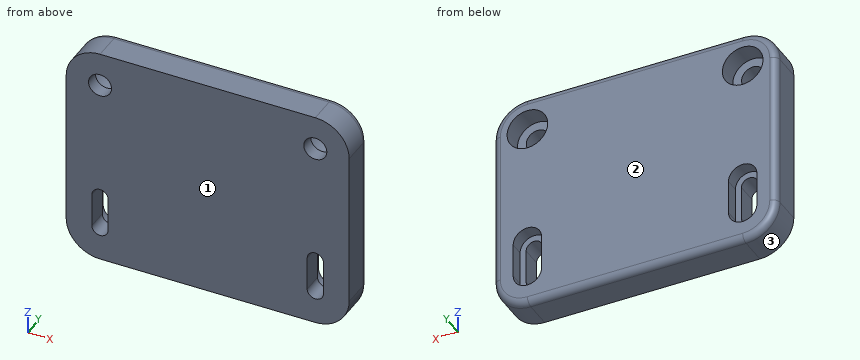
```python
from build123d import *

# Parameters (mm, degrees)
SKETCH1_W           = 41.8
SKETCH1_H           = 33
SKETCH1_R           = 1.7
BOSS_EXTRUDE1_DEPTH = 5
FILLET1_R           = 5
FILLET2_R           = 1
SKETCH2_R           = 3
SKETCH2_R_2         = 1.7
CUT_EXTRUDE1_DEPTH  = 3
CUT_EXTRUDE2_DEPTH  = 2


with BuildPart() as part:
    # Sketch1 → Boss-Extrude1 (new body)
    with BuildSketch(Plane(origin=(0, 0, 0), x_dir=(1, 0, 0), z_dir=(0, 1, 0))):
        with Locations((20.9, 16.5)):
            Rectangle(SKETCH1_W, SKETCH1_H)
        with Locations((5, 5)):
            Circle(SKETCH1_R, mode=Mode.SUBTRACT)
        with Locations((36.8, 5)):
            Circle(SKETCH1_R, mode=Mode.SUBTRACT)
        with BuildLine():
            Line((3.8, 23), (3.8, 28))
            ThreePointArc((3.8, 28), (5, 29.2), (6.2, 28))
            Line((6.2, 28), (6.2, 23))
            ThreePointArc((6.2, 23), (5, 21.8), (3.8, 23))
        make_face(mode=Mode.SUBTRACT)
        with BuildLine():
            Line((35.6, 23), (35.6, 28))
            ThreePointArc((35.6, 28), (36.8, 29.2), (38, 28))
            Line((38, 28), (38, 23))
            ThreePointArc((38, 23), (36.8, 21.8), (35.6, 23))
        make_face(mode=Mode.SUBTRACT)
    extrude(amount=BOSS_EXTRUDE1_DEPTH)

    # Fillet1
    fillet1_edges = [part.edges().sort_by_distance(p)[0] for p in [
        (0, 2.5, -33),
        (41.8, 2.5, -33),
        (41.8, 2.5, 0),
        (0, 2.5, 0),
    ]]
    fillet(fillet1_edges, radius=FILLET1_R)

    # Fillet2
    fillet2_edges = [part.edges().sort_by_distance(p)[0] for p in [
        (0, 5, -16.5),
        (20.9, 5, -33),
        (20.9, 5, 0),
        (41.8, 5, -16.5),
        (1.464466094, 5, -1.464466094),
        (40.335533906, 5, -1.464466094),
        (40.335533906, 5, -31.535533906),
        (1.464466094, 5, -31.535533906),
    ]]
    fillet(fillet2_edges, radius=FILLET2_R)

    # Sketch2 → Cut-Extrude1 (cut)
    with BuildSketch(Plane(origin=(0, 5, 0), x_dir=(1, 0, 0), z_dir=(0, 1, 0))):
        with Locations((5, 5)):
            Circle(SKETCH2_R)
        with Locations((5, 5)):
            Circle(SKETCH2_R_2, mode=Mode.SUBTRACT)
        with Locations((36.8, 5)):
            Circle(SKETCH2_R)
        with Locations((36.8, 5)):
            Circle(SKETCH2_R_2, mode=Mode.SUBTRACT)
    extrude(amount=-CUT_EXTRUDE1_DEPTH, mode=Mode.SUBTRACT)

    # Sketch2_3 → Cut-Extrude2 (cut)
    with BuildSketch(Plane(origin=(0, 5, 0), x_dir=(1, 0, 0), z_dir=(0, 1, 0))):
        with BuildLine():
            Line((2.9, 28), (2.9, 23))
            ThreePointArc((2.9, 23), (5, 20.9), (7.1, 23))
            Line((7.1, 23), (7.1, 28))
            ThreePointArc((7.1, 28), (5, 30.1), (2.9, 28))
        make_face()
        with BuildLine():
            Line((6.2, 28), (6.2, 23))
            ThreePointArc((6.2, 23), (5, 21.8), (3.8, 23))
            Line((3.8, 23), (3.8, 28))
            ThreePointArc((3.8, 28), (5, 29.2), (6.2, 28))
        make_face(mode=Mode.SUBTRACT)
        with BuildLine():
            Line((34.7, 28), (34.7, 23))
            ThreePointArc((34.7, 23), (36.8, 20.9), (38.9, 23))
            Line((38.9, 23), (38.9, 28))
            ThreePointArc((38.9, 28), (36.8, 30.1), (34.7, 28))
        make_face()
        with BuildLine():
            Line((38, 28), (38, 23))
            ThreePointArc((38, 23), (36.8, 21.8), (35.6, 23))
            Line((35.6, 23), (35.6, 28))
            ThreePointArc((35.6, 28), (36.8, 29.2), (38, 28))
        make_face(mode=Mode.SUBTRACT)
    extrude(amount=-CUT_EXTRUDE2_DEPTH, mode=Mode.SUBTRACT)


solid = part.part
```
Build history of the part. All positions in model axes, mm. Face numbers are marked on the shaded views. Round coordinates to 2 decimals unless told otherwise and drop trailing zeros. Write each loop counter-clockwise with the first axis right and the second up, starting at its lowest first coordinate (ties: lowest second). Pieces come first, ordered by that corner, then holes.
1) Drill centre lines: probe 1 along Z at (x, y) = (36.8, 3.65); probe 2 along Z at (x, y) = (5, 1.05); probe 3 along X at (y, z) = (2.35, -28.5). Where is each one in solid material? Low to high.
2) Pin check, flat tip, straight feed: pin 1 (5.5 mm diameter, centred on x = 5, z = -5, fed in from +Y). Stop position of the tip, or through.
3) Mould opens along Y. For the marked faces 1, 2 and 3 say: +Y half, -Y half, draft (parallel to the pull), parting line (faces both ways), or undercut.
4) Band-saw the part on B-B, the plane z = -23.5. List the corners of the cut face in (x, y), and give its area (3 significant figures).
5) Band-saw the part on A-A, the plane y = 1.3. List the corners of the cut face in (x, z).
Ans:
1. probe 1: z = -33 to -30.1, -20.9 to -8, -2 to 0
1. probe 2: z = -33 to -29.2, -21.8 to -6.7, -3.3 to 0
1. probe 3: x = 0.03 to 3.91, 6.09 to 35.71, 37.89 to 41.77
2. pin 1: stops at y = 2
3. face 1: -Y half
3. face 2: +Y half
3. face 3: draft
4. outline: (0, 0) - (3.8, 0) - (3.8, 3) - (2.9, 3) - (2.9, 5) - (1, 5) arc R1 ccw to (0, 4) - close; (6.2, 0) - (35.6, 0) - (35.6, 3) - (34.7, 3) - (34.7, 5) - (7.1, 5) - (7.1, 3) - (6.2, 3) - close; (38, 0) - (41.8, 0) - (41.8, 4) arc R1 ccw to (40.8, 5) - (38.9, 5) - (38.9, 3) - (38, 3) - close
4. area: 177 mm2
5. outline: (0, -28) arc R5 ccw to (5, -33) - (36.8, -33) arc R5 ccw to (41.8, -28) - (41.8, -5) arc R5 ccw to (36.8, 0) - (5, 0) arc R5 ccw to (0, -5) - close; hole circle Ø3.4 at (5, -5); hole (3.8, -28) arc R1.2 ccw to (6.2, -28) - (6.2, -23) arc R1.2 ccw to (3.8, -23) - close; hole circle Ø3.4 at (36.8, -5); hole (35.6, -28) arc R1.2 ccw to (38, -28) - (38, -23) arc R1.2 ccw to (35.6, -23) - close
